Autodesk Inventor part; units mm, degrees
ref_plane "YZ Plane" through (0, 0, 0) normal (1, 0, 0) x (0, 1, 0)
ref_plane "XZ Plane" through (0, 0, 0) normal (0, 1, 0) x (-1, 0, 0)
ref_plane "XY Plane" through (0, 0, 0) normal (0, 0, 1) x (1, 0, 0)
sketch "Sketch6" plane through (0, 0, 0) normal (0, 1, 0) x (-1, 0, 0)
  line L0 (32.5, 62.5) -> (-32.5, 62.5)
  line L1 (-42.5, 52.5) -> (-42.5, -52.5)
  line L2 (-32.5, -62.5) -> (32.5, -62.5)
  line L3 (42.5, -52.5) -> (42.5, 52.5)
  line L4 (42.5, 62.5) -> (-42.5, -62.5) construction
  line L5 (-42.5, 62.5) -> (42.5, -62.5) construction
  circle A0 centre (0, -36.5125) radius 3.25
  circle A1 centre (0, 48.4875) radius 3.25
  arc A2 (32.5, -62.5) -> (42.5, -52.5) centre (32.5, -52.5) ccw
  arc A3 (-42.5, -52.5) -> (-32.5, -62.5) centre (-32.5, -52.5) ccw
  arc A4 (-32.5, 62.5) -> (-42.5, 52.5) centre (-32.5, 52.5) ccw
  arc A5 (42.5, 52.5) -> (32.5, 62.5) centre (32.5, 52.5) ccw
  circle A6 centre (0, 48.4875) radius 5.5
  circle A7 centre (0, -36.5125) radius 5.5
  line L6 (-1.445, 54.6718) -> (4.6332, 52.8311)
  line L7 (4.6332, 52.8311) -> (6.0782, 46.6468)
  line L8 (6.0782, 46.6468) -> (1.445, 42.3032)
  line L9 (1.445, 42.3032) -> (-4.6332, 44.1439)
  line L10 (-4.6332, 44.1439) -> (-6.0782, 50.3282)
  line L11 (-6.0782, 50.3282) -> (-1.445, 54.6718)
  line L12 (-1.445, -30.3282) -> (4.6332, -32.1689)
  line L13 (4.6332, -32.1689) -> (6.0782, -38.3532)
  line L14 (6.0782, -38.3532) -> (1.445, -42.6968)
  line L15 (1.445, -42.6968) -> (-4.6332, -40.8561)
  line L16 (-4.6332, -40.8561) -> (-6.0782, -34.6718)
  line L17 (-6.0782, -34.6718) -> (-1.445, -30.3282)
  point P0 (0, 0)
  point P1 (-3.7616, 52.5)
  point P2 (-3.7616, -32.5)
  dimension "d48" = 11
  dimension "d49" = 11
  dimension "d42" = 85
  dimension "d43" = 125
  dimension "d44" = 6.5
  dimension "d45" = 6.5
  dimension "d46" = 85
  dimension "d47" = 10
extrude "Extrusion6" add sketch "Sketch6" along normal blind 2 contours A5 L3 A2 L2 A3 L1 A4 L0 | A6 | A6 L7 L8 | A6 L6 L7 | L8 L9 A6 | A6 L11 L6 | L9 L10 A6 | A6 L10 L11 | A7 | A7 L13 L14 | A7 L12 L13 | L14 L15 A7 | A7 L17 L12 | L15 L16 A7 | A7 L16 L17
sketch "Sketch7" plane through (0, 2, 0) normal (0, 1, 0) x (1, 0, 0)
  circle A0 centre (0, -48.4875) radius 3.25
  circle A1 centre (0, -48.4875) radius 5.5
  circle A2 centre (0, 36.5125) radius 3.25
  circle A3 centre (0, 36.5125) radius 5.5
  line L0 (5.5, -51.6629) -> (0, -54.8384)
  line L1 (0, -54.8384) -> (-5.5, -51.6629)
  line L2 (-5.5, -51.6629) -> (-5.5, -45.3121)
  line L3 (-5.5, -45.3121) -> (0, -42.1366)
  line L4 (0, -42.1366) -> (5.5, -45.3121)
  line L5 (5.5, -45.3121) -> (5.5, -51.6629)
  line L6 (5.5, 33.3371) -> (0, 30.1616)
  line L7 (0, 30.1616) -> (-5.5, 33.3371)
  line L8 (-5.5, 33.3371) -> (-5.5, 39.6879)
  line L9 (-5.5, 39.6879) -> (0, 42.8634)
  line L10 (0, 42.8634) -> (5.5, 39.6879)
  line L11 (5.5, 39.6879) -> (5.5, 33.3371)
  line L12 (-32.5, 62.5) -> (32.5, 62.5)
  line L13 (42.5, 52.5) -> (42.5, -52.5)
  line L14 (32.5, -62.5) -> (-32.5, -62.5)
  line L15 (-42.5, -52.5) -> (-42.5, 52.5)
  line L16 (-42.5, 62.5) -> (42.5, -62.5) construction
  line L17 (42.5, 62.5) -> (-42.5, -62.5) construction
  arc A4 (-42.5, -52.5) -> (-32.5, -62.5) centre (-32.5, -52.5) ccw
  arc A5 (-32.5, 62.5) -> (-42.5, 52.5) centre (-32.5, 52.5) ccw
  arc A6 (42.5, 52.5) -> (32.5, 62.5) centre (32.5, 52.5) ccw
  arc A7 (32.5, -62.5) -> (42.5, -52.5) centre (32.5, -52.5) ccw
  point P0 (0, 0)
  point P1 (5.5, -48.4875)
  point P2 (5.5, 36.5125)
  dimension "d52" = 11
  dimension "d53" = 11
  dimension "d54" = 125
  dimension "d61" = 10
extrude "Extrusion7" add sketch "Sketch7" along normal blind 3.125 contours L12 A6 L13 A7 L14 A4 L15 A5
sketch "Sketch8" plane through (0, 5.125, 0) normal (0, 1, 0) x (1, 0, 0)
  circle A0 centre (0, -48.4875) radius 3.25
  circle A1 centre (0, -48.4875) radius 3.25
  circle A2 centre (0, 36.5125) radius 3.25
  circle A3 centre (0, 36.5125) radius 3.25
  line L0 (-32.5, 62.5) -> (32.5, 62.5)
  line L1 (42.5, 52.5) -> (42.5, -52.5)
  line L2 (32.5, -62.5) -> (-32.5, -62.5)
  line L3 (-42.5, -52.5) -> (-42.5, 52.5)
  line L4 (-42.5, 62.5) -> (42.5, -62.5) construction
  line L5 (42.5, 62.5) -> (-42.5, -62.5) construction
  arc A4 (32.5, -62.5) -> (42.5, -52.5) centre (32.5, -52.5) ccw
  arc A5 (42.5, 52.5) -> (32.5, 62.5) centre (32.5, 52.5) ccw
  arc A6 (-32.5, 62.5) -> (-42.5, 52.5) centre (-32.5, 52.5) ccw
  arc A7 (-42.5, -52.5) -> (-32.5, -62.5) centre (-32.5, -52.5) ccw
  point P0 (0, 0)
  dimension "d62" = 10
extrude "Extrusion8" add sketch "Sketch8" along normal blind 4.875
sketch "Sketch9" plane through (0, 10, 0) normal (0, 1, 0) x (1, 0, 0)
  line L0 (0, -62.5) -> (0, 62.5)
  line L1 (32.5, 62.5) -> (-32.5, 62.5)
  line L2 (-25, 57.15) -> (-20, 57.15)
  line L3 (-20, 57.15) -> (-20, 12.15)
  line L4 (-20, 12.15) -> (-25, 12.15)
  line L5 (-25, 12.15) -> (-25, 57.15)
  line L6 (32.5, 62.5) -> (-32.5, 62.5)
  line L7 (25, 57.15) -> (20, 57.15)
  line L8 (20, 57.15) -> (20, 12.15)
  line L9 (20, 12.15) -> (25, 12.15)
  line L10 (25, 12.15) -> (25, 57.15)
  point P0 (0, 0)
  dimension "d65" = 5
  dimension "d66" = 45
  dimension "d67" = 20
extrude "Extrusion9" add sketch "Sketch9" along normal blind 60
properties part number "Camera Mount"
The model under review builds one solid part; all positions refer to its coordinate system, in mm. A direction names the side the tool comes from. Round coordinates to 2 decimals unless told otherwise and drop trailing zeros. Loops run counter-clockwise (first coordinate to the right, second up) from the corner with the lowest first, then second, coordinate; pieces in that order, holes last. Notation, with made-up numbers: M -8,52 L 46,52 A10 ccw 46,57 Z; hole C 8.5,17 d9. An arc over 180 degrees is marked long. Write item = value, one per line.
Item 1: Take a section at A-A on y = 42.5. Write out the cut boundary in (x, z).
Return value:
outline = M -25,-57.15 L -20,-57.15 L -20,-12.15 L -25,-12.15 Z; M 20,-57.15 L 25,-57.15 L 25,-12.15 L 20,-12.15 Z
Item 2: Take a section at C-C on z = -51. Write out the cut boundary in (x, y).
Return value:
outline = M -42.5,0 L 42.5,0 L 42.5,10 L 25,10 L 25,70 L 20,70 L 20,10 L -20,10 L -20,70 L -25,70 L -25,10 L -42.5,10 Z
Item 3: Take a section at D-D on x = 31. Write out the cut boundary in (y, z).
Return value:
outline = M 0,-62.5 L 10,-62.5 L 10,62.5 L 0,62.5 Z
Item 4: The part is to be moulded in two halves that separate along X. For faces 5 (the flat face through (-2.712, 3.541, 53.273)), 6 (the cylindrical face through (39.65, 4.93, 59.49)), 7 (the cylindrical face through (-39.49, 4.93, 59.65)), 8 (the flat face through (2.71, 3.54, 43.7)), say which applies: released by +X, released by -X, zero draft, split by the parting line, or undercut.
Return value:
face_5 = undercut
face_6 = released by +X
face_7 = released by -X
face_8 = undercut
Item 5: Machinability: for faces 1 (the flat face through (22, 40, -12.15)), 2 (the flat face through (23, 40, -57.15)), 3 (the flat face through (2.789, 3.541, 53.228)), 4 (the flat face through (-25, 40, -34)), which of the approach directions +Z, -Z, +X, -X, +Y, -Y give a long, thin tool a straight path to every point of the face, cutting with its end or side? Answer none if there is none.
Return value:
face_1 = +Z, +X, -X, +Y
face_2 = -Z, +X, -X, +Y
face_3 = none
face_4 = +Z, -Z, -X, +Y
Item 6: Insertion check: P1, Ø4, axis at x = -23, y = 40, coming from the +Z side; P2, Ø22.5, axis at y = 38, z = -38, coming from the -X side; P3, Ø6, axis at x = -32.5, z = -24.5, coming from the +Y side. Each pin has a flat end and moves straight along its axis. Give the tip position at first contact, or say it passes through.
Return value:
P1 = -12.15
P2 = -25
P3 = 10
Item 7: For line 1 (Z direction, x = 0, y = 7); line 2 (X direction, y = 19, z = -25); line 3 (Y direction, x = 37, z = 9.5), list the stretches that pass through material, from the lowest coordinate up. Write a range as [from, to].
Return value:
line_1 = [-62.5, -39.76], [-33.26, 45.24], [51.74, 62.5]
line_2 = [-25, -20], [20, 25]
line_3 = [0, 10]
Item 8: Take a section at B-B on z = -35. Write out the cut boundary in (x, y) (3 decimals).
Return value:
outline = M -42.5,0 L -2.877,0 L -2.877,2 L -5.5,2 L -5.5,5.125 L -2.877,5.125 L -2.877,10 L -20,10 L -20,70 L -25,70 L -25,10 L -42.5,10 Z; M 2.877,0 L 42.5,0 L 42.5,10 L 25,10 L 25,70 L 20,70 L 20,10 L 2.877,10 L 2.877,5.125 L 5.5,5.125 L 5.5,2 L 2.877,2 Z
